Here's how the part is built. I have some questions about the finished solid (model axes, mm). Face numbers are marked on the shaded views. A direction names the side the tool comes from. Give positions to 0.01 mm unless a question says otherwise; leave off trailing zeros. Loops run counter-clockwise (first coordinate to the right, second up) from the corner with the lowest first, then second, coordinate; pieces in that order, holes last. Notation, with made-up numbers: (83.5, 46) -> (91.5, 46) arc R36 ccw to (91.5, 82) -> close; hole circle Ø7 at (-26.75, 88). An arc over 180 degrees is marked (long way). Answer in a Markdown table with one row per item. Add a question column.
Item 1: For P1, Ø1.5, axis at x = 0, y = 2.5, coming from the -Z side; P2, Ø7.5, axis at y = -7, z = 8, coming from the -X side; P3, Ø6, axis at x = 9.5, z = 7.5, coming from the +Y side, each with a flat end and sliding along its axis, tell me the tip position at first contact or that it passes through.
Item 2: Which directions (+Z, -Z, +X, -X, +Y, -Y) give clear straight access to the entire face, cutting with the end or side of a thin tool? Please do the marked faces 4, 5, 6, 7 and 8.
Item 3: If we section it at A-A (x = -9.5): Write out the boundary of the cut face in (y, z).
Item 4: If we section it at C-C (z = 7.75): Give the number of separate pieces and of enclosed holes in the cut face, then the cut area to 3 significant figures.
Item 5: We'd pull the mould along Z, two halves only. Please class the marked faces 1, 2 and 3: released by +Z, released by -Z, zero draft, split by the parting line, or undercut.
Item 6: If I drill on line 1 (Y direction, x = 12, z = 7.75); line 2 (X direction, y = -7.5, z = 0.8); line 3 (X direction, y = -6.25, z = 2.25), over which ranges is the centre line in solid material (lowest first)?
```python
from build123d import *

# Parameters (mm, degrees)
BOSS_EXTRUDE1_DEPTH = 15.5
FILLET1_R           = 5
SKETCH5_W           = 13
SKETCH5_H           = 9.5
CUT_EXTRUDE3_DEPTH  = 36.29164207
SKETCH6_W           = 5
SKETCH6_H           = 5.5
BOSS_EXTRUDE2_DEPTH = 5
FILLET2_R           = 2.5
FILLET3_R           = 2.5
SKETCH3_R           = 1.65
CUT_EXTRUDE4_DEPTH  = 29.574464179
SKETCH8_R           = 0.75
CUT_EXTRUDE7_DEPTH  = 44.873285276
SKETCH9_R           = 0.75
CUT_EXTRUDE9_DEPTH  = 17.215351852


with BuildPart() as part:
    # Sketch2 → Boss-Extrude1 (new body)
    with BuildSketch(Plane.XY):
        with BuildLine():
            Line((-12.5, 0), (12.5, 0))
            ThreePointArc((12.5, 0), (19.5, -7), (12.5, -14))
            Line((12.5, -14), (-12.5, -14))
            ThreePointArc((-12.5, -14), (-19.5, -7), (-12.5, 0))
        make_face()
    extrude(amount=BOSS_EXTRUDE1_DEPTH)

    # Fillet1
    fillet1_edges = [part.edges().sort_by_distance(p)[0] for p in [
        (-19.5, -7, 15.5),
        (0, -14, 15.5),
        (19.5, -7, 15.5),
        (0, -14, 0),
        (-19.5, -7, 0),
        (0, 0, 0),
        (19.5, -7, 0),
        (0, 0, 15.5),
    ]]
    fillet(fillet1_edges, radius=FILLET1_R)

    # Sketch5 → Cut-Extrude3 (cut, through all)
    with BuildSketch(Plane(origin=(0, -25, 0), x_dir=(-1, 0, 0), z_dir=(0, -1, 0))):
        with Locations((13, -7.75)):
            Rectangle(SKETCH5_W, SKETCH5_H)
    extrude(amount=-CUT_EXTRUDE3_DEPTH, mode=Mode.SUBTRACT)

    # Sketch6 → Boss-Extrude2 (add)
    with BuildSketch(Plane(origin=(0, 0, 0), x_dir=(1, 0, 0), z_dir=(0, 1, 0))):
        with Locations((2, -7.75)):
            Rectangle(SKETCH6_W, SKETCH6_H)
    extrude(amount=BOSS_EXTRUDE2_DEPTH)

    # Fillet2
    fillet2_edges = [part.edges().sort_by_distance(p)[0] for p in [
        (4.5, 5, 7.75),
        (-0.5, 5, 7.75),
    ]]
    fillet(fillet2_edges, radius=FILLET2_R - 0.0001)  # a hair under: the kernel refuses the full size

    # Fillet3
    fillet3_edges = [part.edges().sort_by_distance(p)[0] for p in [
        (-0.5, 0, 7.75),
        (4.5, 0, 7.75),
    ]]
    fillet(fillet3_edges, radius=FILLET3_R)

    # Sketch3 → Cut-Extrude4 (cut, through all)
    with BuildSketch(Plane.XY.offset(15.5)):
        with Locations((-12.5, -7.5)):
            Circle(SKETCH3_R)
        with Locations(Location((12.5, -7.5, 0), (0, 0, 321.484430951))):
            Circle(SKETCH3_R)
    extrude(amount=-CUT_EXTRUDE4_DEPTH, mode=Mode.SUBTRACT)

    # Sketch8 → Cut-Extrude7 (cut, through all)
    with BuildSketch(Plane(origin=(19.5, 0, 0), x_dir=(0, 0, -1), z_dir=(1, 0, 0))):
        with Locations((-7.75, -4)):
            Circle(SKETCH8_R)
    extrude(amount=-CUT_EXTRUDE7_DEPTH, mode=Mode.SUBTRACT)

    # Sketch9 → Cut-Extrude9 (cut, along a direction that is not the sketch's normal)
    with BuildSketch(Plane.ZY.offset(6.5)):
        with Locations((7.75, -10)):
            Circle(SKETCH9_R)
    extrude(amount=-CUT_EXTRUDE9_DEPTH, dir=(-0.9294030199155335, 0.36906642569039866, 0), mode=Mode.SUBTRACT)


solid = part.part
```
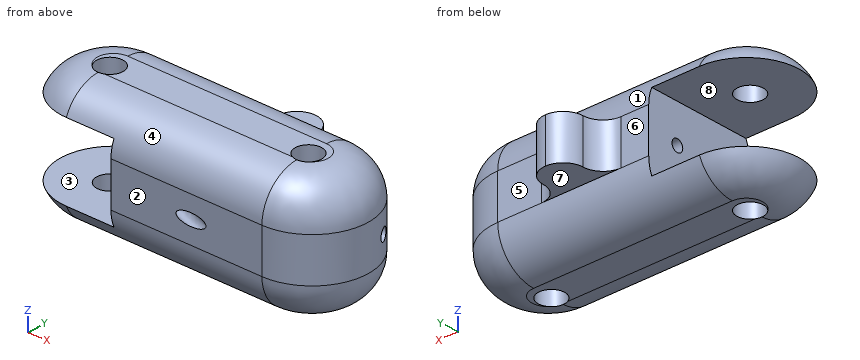
Recorded:
| question | item | result |
|---|---|---|
| 1 | P1 | stops at z = 5 |
| 1 | P2 | stops at x = -6.5 |
| 1 | P3 | stops at y = 0.05 |
| 2 | face 4 | +Z, +X, -X, -Y |
| 2 | face 5 | +Z, -Z, +X, +Y |
| 2 | face 6 | +Z, -Z, -X, +Y |
| 2 | face 7 | -Z, +X, -X, +Y |
| 2 | face 8 | -X, +Y, -Y |
| 3 | outline | (-13.58, 3) arc R5 ccw to (-9, 0) -> (-5, 0) arc R5 ccw to (-0.42, 3) -> close; (-13.58, 12.5) -> (-0.42, 12.5) arc R5 ccw to (-5, 15.5) -> (-9, 15.5) arc R5 ccw to start |
| 4 | separate pieces | 3 |
| 4 | enclosed holes | 1 |
| 4 | area | 306 mm^2 |
| 5 | face 1 | released by +Z |
| 5 | face 2 | zero draft |
| 5 | face 3 | undercut |
| 6 | line 1 | y = -14 to -9.07, -5.93 to -4.75, -3.25 to 0 |
| 6 | line 2 | x = -17.19 to -14.15, -10.85 to 10.85, 14.15 to 17.19 |
| 6 | line 3 | x = -18.63 to -13.58, -11.42 to 11.42, 13.58 to 18.63 |
